from build123d import *

# Parameters (mm, degrees)
CYLINDER015_R          = 21
CYLINDER015_DEPTH      = 25
CYLINDER016_R          = 25
CYLINDER016_DEPTH      = 25
CUT004_ROLL_ANGLE      = 90
CUT004_PITCH_ANGLE     = -7e-06
CUT004_PLACEMENT_ANGLE = -179.999993


with BuildPart() as cylinder015:
    # Cylinder015 → Cylinder015 (new body)
    with BuildSketch(Plane.XY):
        Circle(CYLINDER015_R)
    extrude(amount=CYLINDER015_DEPTH)


with BuildPart() as cut004:
    # Cylinder016 → Cylinder016 (new body)
    with BuildSketch(Plane.XY):
        Circle(CYLINDER016_R)
    extrude(amount=CYLINDER016_DEPTH)

    # Cut004: cut Cylinder015
    add(cylinder015.part, mode=Mode.SUBTRACT)


with BuildPart() as cut004_1:
    # Cut004 roll: moved
    add(cut004.part.rotate(Axis((0, 0, 0), (1, 0, 0)), CUT004_ROLL_ANGLE))


with BuildPart() as cut004_2:
    # Cut004 pitch: moved
    add(cut004_1.part.rotate(Axis((0, 0, 0), (0, 1, 0)), CUT004_PITCH_ANGLE))


with BuildPart() as cut004_3:
    # Cut004 placement: moved
    add(cut004_2.part.moved(Location((22.3, -76, -12))).rotate(Axis((22.3, -76, -12), (0, 0, 1)), CUT004_PLACEMENT_ANGLE))


solid = cut004_3.part
Read the model definition and answer for the solid it produces. Units are mm, in the model's axes. Round coordinates to 2 decimals unless told otherwise and drop trailing zeros. Write each loop counter-clockwise with the first axis right and the second up, starting at its lowest first coordinate (ties: lowest second). Pieces come first, ordered by that corner, then holes.
Q1. Flat-ended cylindrical pins translate along their axes: P1, Ø5, axis at y = -56, z = 7.5, coming from the +X side; P2, Ø12, axis at y = -59, z = -29, coming from the -X side; P3, Ø10, axis at x = 12.5, y = -54, coming from the -Z side; P4, Ø10, axis at x = 5, z = -11.5, coming from the -Y side. Find the tip coordinate at first contact, or state that the pin passes through.
Values:
P1: stops at x = 40.63
P2: stops at x = -0.15
P3: stops at z = -36.53
P4: stops at y = -76
Q2. Find section A-A on z = -29. Determine the outline of the cut face in (x, y), and give its area (3 significant figures).
Values:
outline: (3.97, -76) - (9.97, -76) - (9.97, -51) - (3.97, -51) - close; (34.63, -76) - (40.63, -76) - (40.63, -51) - (34.63, -51) - close
area: 300 mm2
Q3. Straight lines are drawn through the part: line 1 (X direction, y = -69.75, z = -12); line 2 (Z direction, x = 22.3, y = -62); line 3 (Z direction, x = 11, y = -53.25). For each, find the intervals that lie inside material, in ascending order.
Values:
line 1: x = -2.7 to 1.3, 43.3 to 47.3
line 2: z = -37 to -33, 9 to 13
line 3: z = -34.3 to -29.7, 5.7 to 10.3
Q4. Find section B-B on z = -7. Determine the outline of the cut face in (x, y), and give its area (3 significant figures).
Values:
outline: (-2.19, -76) - (1.9, -76) - (1.9, -51) - (-2.19, -51) - close; (42.7, -76) - (46.79, -76) - (46.79, -51) - (42.7, -51) - close
area: 205 mm2
